Autodesk Inventor part; units mm, degrees
ref_plane "YZ Plane" through (0, 0, 0) normal (1, 0, 0) x (0, 1, 0)
ref_plane "XZ Plane" through (0, 0, 0) normal (0, 1, 0) x (-1, 0, 0)
ref_plane "XY Plane" through (0, 0, 0) normal (0, 0, 1) x (1, 0, 0)
sketch "Sketch1" plane through (0, 0, 0) normal (0, 0, 1) x (1, 0, 0)
  line L0 (-11.8119, 27.5254) -> (114.7385, 127.5389)
  line L1 (-13.4704, -0.891) -> (100.5859, -114.9473)
  arc A0 (100.5859, -114.9473) -> (330.4805, -114.9473) centre (215.5332, 0) ccw
  arc A1 (330.4805, 114.9473) -> (114.7385, 127.5389) centre (215.5332, 0) ccw
  line L2 (-15.7492, 32.5074) -> (110.8012, 132.5209)
  arc A2 (339.3763, 114.8628) -> (110.8012, 132.5209) centre (215.5332, 0) ccw
  arc A3 (96.0958, -119.4374) -> (339.3763, -114.8628) centre (215.5332, 0) ccw
  line L3 (96.0958, -119.4374) -> (-17.9605, -5.3811)
  arc A4 (-15.7492, 32.5074) -> (-17.9605, -5.3811) centre (0, 12.5794) ccw
  arc A5 (-11.8119, 27.5254) -> (-13.4704, -0.891) centre (0, 12.5794) ccw
  line L4 (330.4805, 114.9473) -> (334.9706, 110.4572)
  line L5 (330.4805, -114.9473) -> (334.9706, -110.4572)
  line L6 (334.9706, -110.4572) -> (339.3763, -114.8628)
  line L7 (334.9706, 110.4572) -> (339.3763, 114.8628)
  point P0 (0, 0)
  dimension "d4" = 6.35
  dimension "d5" = 6.35
extrude "Extrusion1" add sketch "Sketch1" against normal blind 6.35
properties part number "neck chain"
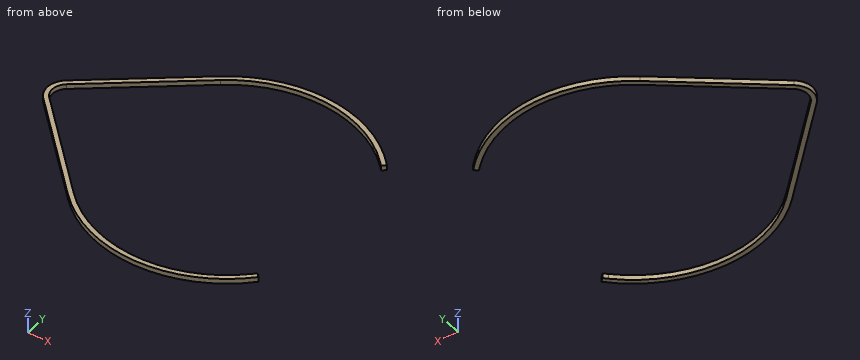
Geometry: final body of the model. Coordinates: model frame, mm. Coordinates: 2 decimals unless noted, no trailing zeros. Order: outer loops, then holes, each group sorted by start corner. A loop starts at its lowest first (then second) coordinate and runs counter-clockwise, first axis right, second up.
(1) Section query D-D (y = 36.5). Return the cut outline in (x, z).
(2) First-contact query: pin 1 (1 mm diameter, centred on y = 93, z = -1, fed in from +X); pin 2 (2 mm diameter, centred on x = 254.5, z = -5, fed in from -Y). Flat tips, straight axial feed; report the tip coordinate or a pass-through.
(3) Section query C-C (x = 191). Return the cut outline in (y, z).
(4) Section query A-A (x = 261). Return the cut outline in (y, z).
(5) Material intervals for probe 1 along X at (y, z) = (146.5, -2); probe 2 along Y at (x, z) = (30.5, -4); probe 3 along Y at (x, z) = (105.5, -3.25), sorted ascending.
(6) Section query B-B (z = -2). Return the cut outline in (x, y).
Solution:
1. outline: (-10.7, -6.35) - (-0.46, -6.35) - (-0.46, 0) - (-10.7, 0) - close
2. pin 1: stops at x = 71.67
2. pin 2: stops at y = -164.59
3. outline: (-167.12, -6.35) - (-160.7, -6.35) - (-160.7, 0) - (-167.12, 0) - close; (160.7, -6.35) - (167.12, -6.35) - (167.12, 0) - (160.7, 0) - close
4. outline: (-162.68, -6.35) - (-156.07, -6.35) - (-156.07, 0) - (-162.68, 0) - close; (156.07, -6.35) - (162.68, -6.35) - (162.68, 0) - (156.07, 0) - close
5. probe 1: x = 131.46 to 145.08, 285.99 to 299.61
5. probe 2: y = -53.84 to -44.86, 60.96 to 69.06
5. probe 3: y = -128.15 to -119.66, 120.24 to 128.33
6. outline: (-17.96, -5.38) - (96.1, -119.44) arc R168.91 ccw to (339.38, -114.86) - (334.97, -110.46) - (330.48, -114.95) arc R162.56 cw to (100.59, -114.95) - (-13.47, -0.89) arc R19.05 cw to (-11.81, 27.53) - (114.74, 127.54) arc R162.56 cw to (330.48, 114.95) - (334.97, 110.46) - (339.38, 114.86) arc R168.91 ccw to (110.8, 132.52) - (-15.75, 32.51) arc R25.4 ccw to start
